Study the drawing (mm; zero at the part's minimum x, y, z) and answer. Round coordinates to 2 decimals unless told otherwise and drop trailing zeros. Write each loop counter-clockwise with the first axis right and the second up, starting at its lowest first coordinate (ties: lowest second). Pieces come first, ordered by that corner, then holes.
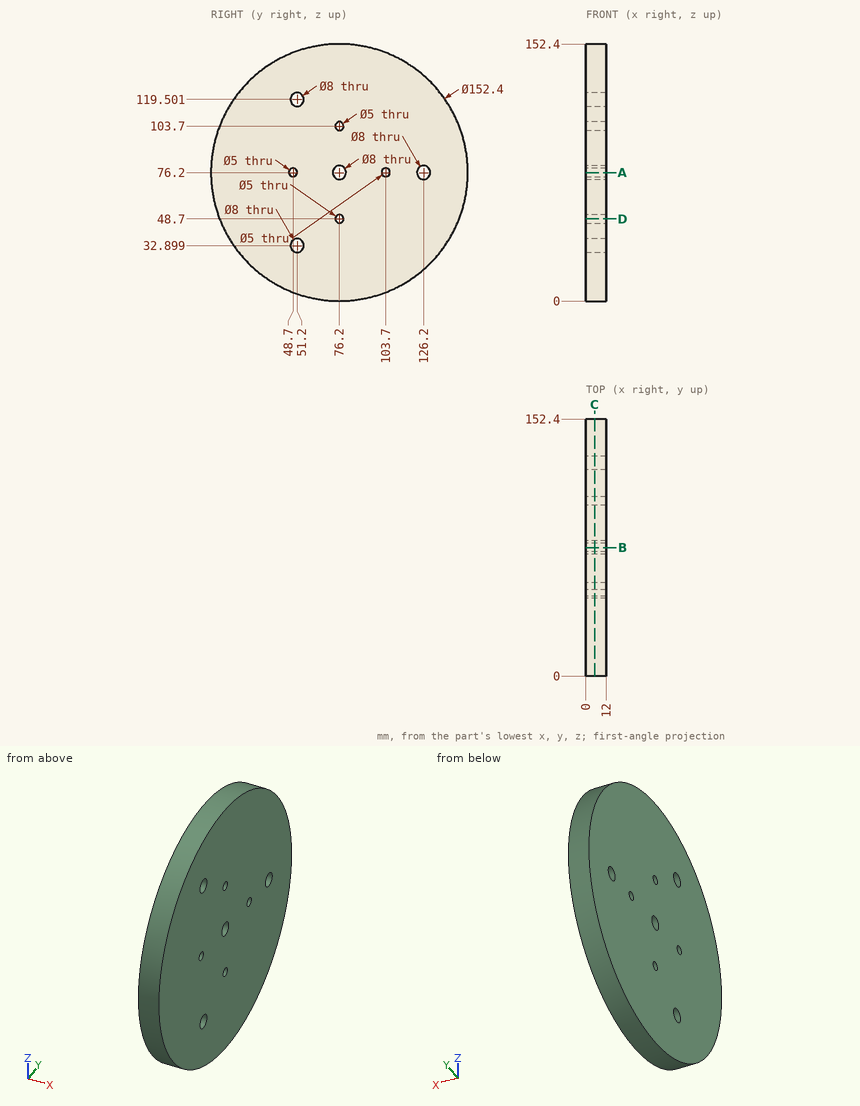
1. Given pin 1 (6.5 mm diameter, centred on y = 76.2, z = 76.2, fed in from -X); pin 2 (4 mm diameter, centred on x = 7.5, y = 120.5, fed in from -Z); pin 3 (1.5 mm diameter, centred on x = 7.5, y = 129, fed in from -Z); pin 4 (5 mm diameter, centred on x = 8.5, z = 43.5, fed in from +Y), each flat-ended and moving along its own axis, determine where each tip first touches the part or whether it passes through.
Geometry says:
pin 1: passes through
pin 2: stops at z = 12.82
pin 3: stops at z = 20.55
pin 4: stops at y = 146.16
2. Section A-A on z = 76.2 is taken. Determine the outline of the cut face in (x, y).
Geometry says:
outline: (0, 0) - (12, 0) - (12, 46.2) - (0, 46.2) - close; (0, 51.2) - (12, 51.2) - (12, 72.2) - (0, 72.2) - close; (0, 80.2) - (12, 80.2) - (12, 101.2) - (0, 101.2) - close; (0, 106.2) - (12, 106.2) - (12, 122.2) - (0, 122.2) - close; (0, 130.2) - (12, 130.2) - (12, 152.4) - (0, 152.4) - close
3. Section B-B on y = 76.2 is taken. Determine the outline of the cut face in (x, z).
Geometry says:
outline: (0, 0) - (12, 0) - (12, 46.2) - (0, 46.2) - close; (0, 51.2) - (12, 51.2) - (12, 72.2) - (0, 72.2) - close; (0, 80.2) - (12, 80.2) - (12, 101.2) - (0, 101.2) - close; (0, 106.2) - (12, 106.2) - (12, 152.4) - (0, 152.4) - close
4. Section D-D on z = 48.7 is taken. Determine the outline of the cut face in (x, y) (1 decimal), plus the area to 3 significant figures.
Geometry says:
outline: (0, 5.1) - (12, 5.1) - (12, 73.7) - (0, 73.7) - close; (0, 78.7) - (12, 78.7) - (12, 147.3) - (0, 147.3) - close
area: 1,650 mm2
5. Section C-C on x = 5.25 is taken. Give the number of separate pieces and of enclosed holes in the cut face, plus the area to 3 significant figures.
Geometry says:
separate pieces: 1
enclosed holes: 8
area: 18,000 mm2
6. Straight lines are drawn through the part: line 1 along Y through (x, z) = (3.5, 76.2); line 2 along Y through (x, z) = (11.25, 74) (1 decimal); line 3 along Z through (x, y) = (9, 50) (1 decimal). For each, find the intervals that lie inside material, in ascending order.
Geometry says:
line 1: y = 0 to 46.2, 51.2 to 72.2, 80.2 to 101.2, 106.2 to 122.2, 130.2 to 152.4
line 2: y = 0 to 47.5, 49.9 to 72.9, 79.5 to 102.5, 104.9 to 122.9, 129.5 to 152.4
line 3: z = 4.6 to 29.1, 36.7 to 74.1, 78.3 to 115.7, 123.3 to 147.8
